Work out the finished part from the listing and answer in its coordinate system (mm). A direction names the side the tool comes from. Coordinates: 2 decimals unless noted, no trailing zeros. Loops run counter-clockwise (first coordinate to the right, second up) from the corner with the lowest first, then second, coordinate; pieces in that order, holes last. Notation, with made-up numbers: (61.25, 70.25) - (96.25, 70.25) arc R20 cw to (96.25, 95.25) - close; hole circle Ø1 at (85.5, -34.5). An arc over 180 degrees is marked (long way). Write each question's results on one line, items separated by ' | '. Start each with the question number.
Item 1: Section C-C, the plane y = 28 is taken. Write down the section's boundary in (x, z).
Item 2: Section B-B, the plane z = 57.5 is taken. Write down the section's boundary in (x, y), plus the area to 3 significant figures.
Item 3: For a pull along X with two mould halves and no side action, classify faces 3 (the face through (2.217, 8.113, 44.321)), 4 (the face through (3.4, 25, 44)), 5 (the face through (0, 49, 44)), 6 (the face through (2, 26.15, 44)) as +X half, -X half, draft (parallel to the pull), parting line (faces both ways), or undercut.
Item 4: Each of these flat-tipped pins is pushed along its axis until it touches: pin 1 Ø0.7 at (x, z) = (1.5, 51.5) entering from -Y; pin 2 Ø1 at (x, z) = (2, 66.5) entering from -Y; pin 3 Ø2 at (x, z) = (2.5, 76.5) entering from +Y. Where does it stop, or does it pass through?
Item 5: Consider probe 1 along Y at (x, z) = (2.9, 82); probe 2 along Y at (x, z) = (1.1, 9); probe 3 along X at (y, z) = (55.5, 81.5). Determine where each line is inside the solid, lowest interval first. Write a range as [from, to].
Item 6: A tool of negligible diameter and unlimited length cuts with its end or side. For faces 1 (the face through (2, 73.95, 44)), 2 (the face through (3.4, 95, 44)), from which of +Z, -Z, +X, -X, +Y, -Y can it reach the whole face along a straight path? Write none if from no direction.
Item 7: Section A-A, the plane x = 1.8 is taken. Write down the section's boundary in (y, z).
Autodesk Inventor part; units mm, degrees
ref_plane "Work Plane1" through (0, 0, 90) normal (0, 0, -1) x (0, 1, 0)
ref_plane "YZ Plane" through (0, 0, 0) normal (1, 0, 0) x (0, 1, 0)
ref_plane "XZ Plane" through (0, 0, 0) normal (0, 1, 0) x (-1, 0, 0)
sketch "Sketch1" plane through (0, 0, 0) normal (0, 0, 1) x (1, 0, 0)
  line L0 (0, 0) -> (0, 100)
  line L1 (0, 100) -> (1, 100)
  line L2 (1, 100) -> (1, 97.5)
  line L3 (1, 97.5) -> (3.5, 99)
  line L4 (3.5, 99) -> (3.5, 91)
  line L5 (3.5, 91) -> (1, 92.5)
  line L6 (1, 92.5) -> (1, 7.5)
  line L7 (1, 7.5) -> (3.5, 9)
  line L8 (3.5, 9) -> (3.5, 1)
  line L9 (3.5, 1) -> (1, 2.5)
  line L10 (1, 2.5) -> (1, 0)
  line L11 (1, 0) -> (0, 0)
  line L12 (1, 76.25) -> (3.5, 76.25)
  line L13 (3.5, 76.25) -> (3.5, 73.75)
  line L14 (3.5, 73.75) -> (1, 73.75)
  line L15 (1, 73.75) -> (1, 76.25)
  line L16 (1, 23.75) -> (3.5, 23.75)
  line L17 (3.5, 23.75) -> (3.5, 26.25)
  line L18 (3.5, 26.25) -> (1, 26.25)
  line L19 (1, 26.25) -> (1, 23.75)
  line L20 (3.4, 98.8234) -> (0.9, 97.3234)
  line L21 (0.9, 97.3234) -> (0.9, 99.9)
  line L22 (0.9, 99.9) -> (0.1, 99.9)
  line L23 (0.1, 99.9) -> (0.1, 0.1)
  line L24 (0.1, 0.1) -> (0.9, 0.1)
  line L25 (0.9, 0.1) -> (0.9, 2.6766)
  line L26 (0.9, 2.6766) -> (3.4, 1.1766)
  line L27 (3.4, 1.1766) -> (3.4, 8.8234)
  line L28 (3.4, 8.8234) -> (0.9, 7.3234)
  line L29 (0.9, 7.3234) -> (0.9, 92.6766)
  line L30 (0.9, 92.6766) -> (3.4, 91.1766)
  line L31 (3.4, 91.1766) -> (3.4, 98.8234)
  line L32 (1, 92.5) -> (1, 97.5)
  line L33 (1, 2.5) -> (1, 7.5)
  point P0 (1, 98.75)
  point P1 (0.5, 0)
  point P2 (3.5, 75)
  point P3 (3.5, 25)
  point P4 (1, 97.3834)
  point P5 (1, 92.6166)
  point P6 (1, 7.3834)
  point P7 (1, 2.6166)
  dimension "d0" = 8
  dimension "d1" = 8
  dimension "d2" = 2.5
  dimension "d3" = 2.5
  dimension "d4" = 1
  dimension "d5" = 1
  dimension "d6" = 100
  dimension "d7" = 5
  dimension "d8" = 5
  dimension "d10" = 2.5
  dimension "d11" = 7.5
  dimension "d12" = 2.5
  dimension "d13" = 1
  dimension "d16" = 2.5
  dimension "d17" = 2.5
  dimension "d18" = 2.5
  dimension "d19" = 2.5
  dimension "d20" = 25
  dimension "d21" = 25
  dimension "d24" = 0.1
extrude "Extrusion1" add sketch "Sketch1" along normal blind 90 contours L0 L1 L2 L32 L20 L21 L22 L23 L24 L25 L26 L33 L10 L11 | L33 L26 L27 L28 L7 L8 L9 | L3 L4 L5 L32 L30 L31 L20 | L33 L28 L27 L26 | L26 L25 L24 L23 L22 L21 L20 L32 L30 L29 L28 L33 | L20 L31 L30 L32 | L28 L29 L30 L32 L6 L33
extrude "Extrusion2" add sketch "Sketch1" along normal blind 90 contours L6 L18 L17 L16 | L12 L13 L14 L6
ref_plane "Work Plane1" through (0, 0, 90) normal (0, 0, -1) x (0, 1, 0)
extrude "Extrusion3" cut sketch "Sketch1" along normal up to surface (90 mm away) contours L33 L26 L27 L28 L7 L8 L9 | L3 L4 L5 L32 L30 L31 L20
sketch "Sketch2" plane through (0, 0, 90) normal (0, 0, 1) x (1, 0, 0)
  point P0 (0, 0)
sketch "Sketch3" plane through (0, 0, 90) normal (0, 0, 1) x (1, 0, 0)
  line L0 (1, 97.3834) -> (1, 100)
  line L1 (1, 100) -> (0, 100)
  line L2 (0, 100) -> (0, 0)
  line L3 (0, 0) -> (1, 0)
  line L4 (1, 0) -> (1, 2.6166)
  line L5 (1, 2.6166) -> (3.4, 1.1766)
  line L6 (3.4, 1.1766) -> (3.4, 8.8234)
  line L7 (3.4, 8.8234) -> (1, 7.3834)
  line L8 (1, 7.3834) -> (1, 23.75)
  line L9 (1, 23.75) -> (3.5, 23.75)
  line L10 (3.5, 23.75) -> (3.5, 26.25)
  line L11 (3.5, 26.25) -> (1, 26.25)
  line L12 (1, 26.25) -> (1, 73.75)
  line L13 (1, 73.75) -> (3.5, 73.75)
  line L14 (3.5, 73.75) -> (3.5, 76.25)
  line L15 (3.5, 76.25) -> (1, 76.25)
  line L16 (1, 76.25) -> (1, 92.6166)
  line L17 (1, 92.6166) -> (3.4, 91.1766)
  line L18 (3.4, 91.1766) -> (3.4, 98.8234)
  line L19 (3.4, 98.8234) -> (1, 97.3834)
extrude "Extrusion4" cut sketch "Sketch3" against normal blind 0.1
sketch "Sketch4" plane through (0, 0, 0) normal (0, 0, -1) x (-1, 0, 0)
  line L0 (-3.5, 76.25) -> (-1, 76.25)
  line L1 (-3.5, 73.75) -> (-3.5, 76.25)
  line L2 (-1, 73.75) -> (-3.5, 73.75)
  line L3 (-3.5, 26.25) -> (-1, 26.25)
  line L4 (-3.5, 23.75) -> (-3.5, 26.25)
  line L5 (-1, 23.75) -> (-3.5, 23.75)
  line L6 (-1, 76.05) -> (-3.3, 76.05)
  line L7 (-3.3, 76.05) -> (-3.3, 73.95)
  line L8 (-3.3, 73.95) -> (-1, 73.95)
  line L9 (-1, 26.15) -> (-3.4, 26.15)
  line L10 (-3.4, 26.15) -> (-3.4, 23.85)
  line L11 (-3.4, 23.85) -> (-1, 23.85)
  line L12 (-1, 76.25) -> (-1, 73.75)
  line L13 (-1, 26.25) -> (-1, 23.75)
  point P0 (0, 0)
  dimension "d29" = 0.2
  dimension "d30" = 0.1
extrude "Extrusion5" cut sketch "Sketch4" against normal through all contours L0 L12 L6 L7 L8 L2 L1 | L3 L13 L9 L10 L11 L5 L4
equation "\"d27\" = d30"
equation "\"d29\" = 2 * tol"
equation "\"d30\" = tol"
equation "\"tol\" = 0.1"
properties part number "side"
Answer key:
1) outline: (0, 0) - (1, 0) - (1, 89.9) - (0, 89.9) - close
2) outline: (0, 0) - (1, 0) - (1, 2.62) - (3.4, 1.18) - (3.4, 8.82) - (1, 7.38) - (1, 23.85) - (3.4, 23.85) - (3.4, 26.15) - (1, 26.15) - (1, 73.95) - (3.3, 73.95) - (3.3, 76.05) - (1, 76.05) - (1, 92.62) - (3.4, 91.18) - (3.4, 98.82) - (1, 97.38) - (1, 100) - (0, 100) - close | area: 140 mm^2
3) face 3: undercut | face 4: +X half | face 5: -X half | face 6: draft
4) pin 1: stops at y = 2.11 | pin 2: stops at y = 1.72 | pin 3: stops at y = 98.82
5) probe 1: y = [1.48, 8.52], [23.85, 26.15], [73.95, 76.05], [91.48, 98.52] | probe 2: y = [2.56, 7.44], [23.85, 26.15], [73.95, 76.05], [92.56, 97.44] | probe 3: x = [0, 1]
6) face 1: +Z, -Z, +X | face 2: +Z, -Z, +X, +Y, -Y
7) outline: (2.14, 0) - (7.86, 0) - (7.86, 89.9) - (2.14, 89.9) - close; (23.85, 0) - (26.15, 0) - (26.15, 89.9) - (23.85, 89.9) - close; (73.95, 0) - (76.05, 0) - (76.05, 89.9) - (73.95, 89.9) - close; (92.14, 0) - (97.86, 0) - (97.86, 89.9) - (92.14, 89.9) - close
